Check sheet for the modelled part. Datum: model origin and axes. Units: mm. Round coordinates to 2 decimals unless told otherwise and drop trailing zeros. Order: outer loops, then holes, each group sorted by start corner. A loop starts at its lowest first (then second) coordinate and runs counter-clockwise, first axis right, second up. Notation, with made-up numbers: (-11, 16) -> (28, 16) arc R26 cw to (28, 49) -> close; hole circle Ø7 at (83, 10). An arc over 180 degrees is marked (long way). Answer in a Markdown table with one row per item.
from build123d import *

# Parameters (mm, degrees)
SKIZZE1_R                       = 131
SKIZZE1_W                       = 40
SKIZZE1_H                       = 40
AUFSATZ_LINEAR_AUSTRAGEN1_DEPTH = 10
SKIZZE2_W                       = 15.161428906
SKIZZE2_H                       = 7.514920765
SCHNITT_LINEAR_AUSTRAGEN1_DEPTH = 186.531668456
FASE1_SIZE                      = 1


with BuildPart() as part:
    # Skizze1 → Aufsatz-Linear austragen1 (new body)
    with BuildSketch(Plane(origin=(0, 0, 0), x_dir=(1, 0, 0), z_dir=(0, 1, 0))):
        with Locations(Location((0, 0, 0), (0, 0, 270))):
            Circle(SKIZZE1_R)
        Rectangle(SKIZZE1_W, SKIZZE1_H, mode=Mode.SUBTRACT)
    extrude(amount=AUFSATZ_LINEAR_AUSTRAGEN1_DEPTH)

    # Skizze2 → Schnitt-Linear austragen1 (cut, through all)
    with BuildSketch(Plane(origin=(0, 0, 0), x_dir=(1, 0, 0), z_dir=(0, 1, 0))):
        with Locations((0, -129.62528039)):
            Rectangle(SKIZZE2_W, SKIZZE2_H)
    extrude(amount=SCHNITT_LINEAR_AUSTRAGEN1_DEPTH, mode=Mode.SUBTRACT)

    # Skizze4 → Schnitt-Rotation2 (revolve, cut)
    with BuildSketch(Plane(origin=(0, 0, 0), x_dir=(0, 0, -1), z_dir=(1, 0, 0))):
        Polygon((131, 8), (130, 8), (130, 2), (131, 2), (133.611882568, 2), (133.611882568, 8), align=None)
    revolve(axis=Axis((0, 0, 0), (0, 1, 0)), mode=Mode.SUBTRACT)

    # Fase1
    fase1_edges = [part.edges().sort_by_distance(p)[0] for p in [
        (0, 8, -131),
        (0, 2, -131),
    ]]
    chamfer(fase1_edges, length=FASE1_SIZE - 0.0001)  # a hair under: the kernel refuses the full size


solid = part.part
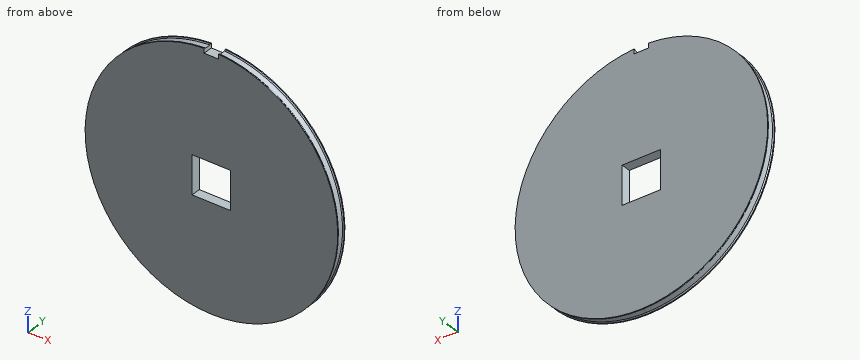
Item 1: Depth check by flat-ended pin: P1, Ø1.5, axis at x = 80, y = 3.5, coming from the -Z side. Enter the tip coordinate at first touch or a pass-through.
Result sheet:
| item | result |
|---|---|
| P1 | stops at z = -103.05 |
Item 2: Cross-section at A-A (y = 4.25). Record the boundary of the cut face in (x, z).
Result sheet:
| item | result |
|---|---|
| outline | (-7.58, 125.87) -> (-7.58, 129.78) arc R130 ccw (long way) to (7.58, 129.78) -> (7.58, 125.87) -> close; hole (-20, -20) -> (20, -20) -> (20, 20) -> (-20, 20) -> close |
Item 3: Scan lines: line 1 (X direction, y = 4.5, z = -2); line 2 (X direction, y = 0.75, z = -17.5); line 3 (X direction, y = 4.75, z = 77). Record each from-to range of solid material in increasing order. Write a range as [from, to].
Result sheet:
| item | result |
|---|---|
| line 1 | x = [-129.98, -20], [20, 129.98] |
| line 2 | x = [-129.83, -20], [20, 129.83] |
| line 3 | x = [-104.74, 104.74] |
